```python
from build123d import *

# Parameters (mm, degrees)
SKETCH2_R = 0.635


with BuildPart() as part:
    # Sweep1: sweep along a path in Sketch1
    with BuildLine(Plane(origin=(0, 0, 0), x_dir=(0, 0, -1), z_dir=(1, 0, 0))) as sweep1_path:
        Line((-2.403997938, -15.816263763), (-0.530715835, -19.857293072))
        ThreePointArc((-0.530715835, -19.857293072), (1.218329614, -21.26591989), (3.400020828, -20.73336666))
        ThreePointArc((3.400020828, -20.73336666), (5.25921097, -17.161895627), (4.04844554, -13.321838283))
        Line((4.04844554, -13.321838283), (1.148017974, -9.865243311))
        ThreePointArc((1.148017974, -9.865243311), (0.295927809, -8.389379852), (0, -6.71108985))
        add(Edge.make_bspline(
            [(0, -6.71108985), (0, 0)],
            knots=[0, 0, 1, 1], degree=1))
    # Sketch2 → Sweep1 (sweep)
    with BuildSketch(Plane(origin=(0, 0, 0), x_dir=(1, 0, 0), z_dir=(0, 1, 0))):
        Circle(SKETCH2_R)
    sweep(path=sweep1_path.line)


solid = part.part
```
Could you check a few things on this model? Use its own coordinates, in mm. Coordinates: 2 decimals unless noted, no trailing zeros. Write item = value, one per line. Start each with the question number.
(1) We'd pull the mould along Y, two halves only. Please class faces 1 (the face through (0, 0, 0)), 2 (the face through (-0.083, -11.165, -3.06)): released by +Y, released by -Y, zero draft, split by the parting line, or undercut.
(2) I need wall thicknesses on line 1 (Z direction, x = 0.05, y = -19.5); line 2 (Y direction, x = -0.1, z = -1.5); line 3 (Z direction, x = 0.45, y = -17.75). Which ranges of each line are inside material? Lowest first, please. Write a range as [from, to].
(3) Will this pin go through, and if not, where does the flat tip stop? pin 1 (3 mm diameter, centred on y = -7, z = 0.5, fed in from -X) (3 decimals).
Result set:
q1.face_1 = released by +Y
q1.face_2 = undercut
q2.line_1 = [-5.21, -3.71], [0, 1.39]
q2.line_2 = [-21.94, -20.68], [-11.26, -9.3]
q2.line_3 = [-5.63, -4.72], [1.01, 2]
q3.pin_1 = -0.635
